Part model, mm, in its own coordinate system. Face numbers are marked on the shaded views. A direction names the side the tool comes from. Give positions to 0.01 mm unless a question says otherwise; leave off trailing zeros. Order: outer loops, then holes, each group sorted by start corner. A loop starts at its lowest first (then second) coordinate and runs counter-clockwise, first axis right, second up.
1. Drop flat-ended pins along their axis: pin 1 Ø8 at (x, z) = (-6.5, 23) entering from +Y; pin 2 Ø6 at (y, z) = (2, 25.5) entering from +X; pin 3 Ø3 at (y, z) = (14.5, 33) entering from +X; pin 4 Ø4 at (x, y) = (9, 14) entering from +Z. Give the stop position or say it passes through.
2. Slice it at B-B on y = 0. List the corners of the cut face in (x, z), and give its area (3 significant figures).
3. Probe line 1 (Y direction, x = 0, z = 15); line 2 (X direction, y = 11, z = 21); line 3 (X direction, y = 4, z = 4.5). List the from-to ranges inside material, lowest first.
4. Mould opens along Y. For the marked faces 6, 7 and 8 say: +Y half, -Y half, draft (parallel to the pull), parting line (faces both ways), or undercut.
5. Slice it at D-D on x = -34. List the corners of the cut face in (y, z).
6. Slice it at A-A on x = 0. List the corners of the cut face in (y, z).
7. Which spindle directions (+Z, -Z, +X, -X, +Y, -Y) get a long thin tool onto all of the face, cutting with end or side? Do the marked faces 1, 2, 3, 4 and 5. Say none if no direction does.
from build123d import *

# Parameters (mm, degrees)
F0_R     = 10
F1_DEPTH = 20
F2_DEPTH = 40
F3_SIZE  = 19.99999


# Not quite as in the source:
# - a fillet or chamfer is up to 0.001 mm smaller than in the source, because OpenCascade refuses the exact size


with BuildPart() as f1:
    # F0 (on Top) → F1 (new body)
    with BuildSketch(Plane.XY):
        with BuildLine():
            Line((15, 20), (-20, 20))
            Line((-20, 20), (-20, 10))
            Line((-20, 10), (-40, 10))
            Line((-40, 10), (-40, -10))
            Line((-40, -10), (-20, -10))
            Line((-20, -10), (-20, -20))
            Line((-20, -20), (15, -20))
            ThreePointArc((15, -20), (18.5355339059, -18.5355339059), (20, -15))
            Line((20, -15), (20, 15))
            ThreePointArc((20, 15), (18.5355339059, 18.5355339059), (15, 20))
        make_face()
        Circle(F0_R, mode=Mode.SUBTRACT)
    extrude(amount=F1_DEPTH)

    # F0 (on Top) → F2 (join)
    with BuildSketch(Plane.XY):
        Polygon((-40, 20), (-50, 20), (-50, 10), (-50, -10), (-50, -20), (-40, -20), (-20, -20), (-20, -10), (-40, -10), (-40, 10), (-20, 10), (-20, 20), align=None)
    extrude(amount=F2_DEPTH)

    # F3 (size 20 in the source; OpenCascade refuses exactly that, so slightly less here)
    f3_edges = [f1.edges().sort_by_distance(p)[0] for p in [
        (-20, -15, 40),
    ]]
    chamfer(f3_edges, length=F3_SIZE)


solid = f1.part
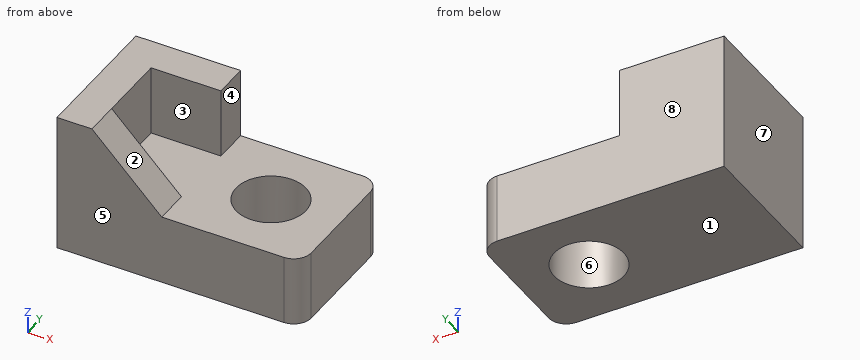
Data:
1. pin 1: stops at y = 20
1. pin 2: stops at x = -40
1. pin 3: stops at x = -20
1. pin 4: stops at z = 20
2. outline: (-50, 0) - (-10, 0) - (-10, 20) - (-40, 20) - (-40, 40) - (-50, 40) - close; (10, 0) - (20, 0) - (20, 20) - (10, 20) - close
2. area: 1,200 mm2
3. line 1: y = -20 to -10, 10 to 20
3. line 2: x = -50 to -20
3. line 3: x = -50 to -9.17, 9.17 to 20
4. face 6: undercut
4. face 7: draft
4. face 8: +Y half
5. outline: (-20, 0) - (20, 0) - (20, 40) - (10, 40) - (10, 20) - (-10, 20) - (-10, 34) - (-20, 34) - close
6. outline: (-20, 0) - (-10, 0) - (-10, 20) - (-20, 20) - close; (10, 0) - (20, 0) - (20, 20) - (10, 20) - close
7. face 1: -Z, +X, -X, +Y, -Y
7. face 2: +Z, +X, -Y
7. face 3: +Z, +X
7. face 4: +Z, +X, +Y, -Y
7. face 5: +Z, -Z, +X, -X, -Y
